Source: CAD feature listing. Evaluate the final solid. Frame: model axes, mm. A direction names the side the tool comes from. Give positions to 0.01 mm unless a question says otherwise; leave off trailing zeros. Loops run counter-clockwise (first coordinate to the right, second up) from the corner with the lowest first, then second, coordinate; pieces in that order, holes last. Notation, with made-up numbers: (-18.75, 40.25) - (-5.75, 40.25) arc R32 ccw to (-5.75, 74.25) - close; hole circle Ø5 at (-40, 25.5). An arc over 180 degrees is marked (long way). Put each result on its own line as item: value.
```python
from build123d import *

# Parameters (mm, degrees)
SKETCH2_W           = 150
SKETCH2_H           = 78
SKETCH2_W_2         = 66
SKETCH2_H_2         = 31
BOSS_EXTRUDE1_DEPTH = 7
FILLET1_R           = 3
SKETCH3_R           = 2.05
CUT_EXTRUDE1_DEPTH  = 10


with BuildPart() as part:
    # Sketch2 → Boss-Extrude1 (new body)
    with BuildSketch(Plane(origin=(0, 0, 0), x_dir=(1, 0, 0), z_dir=(0, 1, 0))):
        Rectangle(SKETCH2_W, SKETCH2_H)
        Rectangle(SKETCH2_W_2, SKETCH2_H_2, mode=Mode.SUBTRACT)
        with BuildLine():
            Line((-39, 10.6), (-36, 10.6))
            ThreePointArc((-36, 10.6), (-33.9, 8.5), (-36, 6.4))
            Line((-36, 6.4), (-39, 6.4))
            ThreePointArc((-39, 6.4), (-41.1, 8.5), (-39, 10.6))
        make_face(mode=Mode.SUBTRACT)
        with BuildLine():
            Line((-39, -10.6), (-36, -10.6))
            ThreePointArc((-36, -10.6), (-33.9, -8.5), (-36, -6.4))
            Line((-36, -6.4), (-39, -6.4))
            ThreePointArc((-39, -6.4), (-41.1, -8.5), (-39, -10.6))
        make_face(mode=Mode.SUBTRACT)
        with BuildLine():
            Line((39, -10.6), (36, -10.6))
            ThreePointArc((36, -10.6), (33.9, -8.5), (36, -6.4))
            Line((36, -6.4), (39, -6.4))
            ThreePointArc((39, -6.4), (41.1, -8.5), (39, -10.6))
        make_face(mode=Mode.SUBTRACT)
        with BuildLine():
            Line((39, 10.6), (36, 10.6))
            ThreePointArc((36, 10.6), (33.9, 8.5), (36, 6.4))
            Line((36, 6.4), (39, 6.4))
            ThreePointArc((39, 6.4), (41.1, 8.5), (39, 10.6))
        make_face(mode=Mode.SUBTRACT)
    extrude(amount=BOSS_EXTRUDE1_DEPTH)

    # Fillet1
    fillet1_edges = [part.edges().sort_by_distance(p)[0] for p in [
        (75, 3.5, 39),
        (-75, 3.5, 39),
        (-75, 3.5, -39),
        (75, 3.5, -39),
    ]]
    fillet(fillet1_edges, radius=FILLET1_R)

    # Sketch3 → Cut-Extrude1 (cut)
    with BuildSketch(Plane(origin=(0, 7, 0), x_dir=(1, 0, 0), z_dir=(0, 1, 0))):
        with Locations(Location((-65, 10, 0), (0, 0, 270))):
            Circle(SKETCH3_R)
        with Locations(Location((-65, 29, 0), (0, 0, 270))):
            Circle(SKETCH3_R)
        with Locations(Location((-65, -10, 0), (0, 0, 270))):
            Circle(SKETCH3_R)
        with Locations(Location((-65, -29, 0), (0, 0, 270))):
            Circle(SKETCH3_R)
        with Locations(Location((65, -29, 0), (0, 0, 270))):
            Circle(SKETCH3_R)
        with Locations(Location((65, -10, 0), (0, 0, 270))):
            Circle(SKETCH3_R)
        with Locations(Location((65, 10, 0), (0, 0, 270))):
            Circle(SKETCH3_R)
        with Locations(Location((65, 29, 0), (0, 0, 270))):
            Circle(SKETCH3_R)
    extrude(amount=-CUT_EXTRUDE1_DEPTH, mode=Mode.SUBTRACT)


solid = part.part
```
1) Material intervals for line 1 along X through (y, z) = (5.75, -29); line 2 along Z through (x, y) = (6, 1); line 3 along X through (y, z) = (6.25, -3), sorted ascending. Write a range as [from, to].
Check result:
line 1: [-75, -67.05], [-62.95, 62.95], [67.05, 75]
line 2: [-39, -15.5], [15.5, 39]
line 3: [-75, -33], [33, 75]
2) Section query C-C, the plane x = -25. Output: boundary loops of the cut face in (y, z).
Check result:
outline: (0, -39) - (7, -39) - (7, -15.5) - (0, -15.5) - close; (0, 15.5) - (7, 15.5) - (7, 39) - (0, 39) - close
3) Pin query (flat end, axial travel): P1, Ø6.5, axis at x = -65, z = 10, coming from the -Y side. Return the tip coordinate at first contact, or that it passes through.
Check result:
P1: y = 0
4) Access query for faces 1 (the flat face through (-33, 3, 0)), 2 (the flat face through (-1, 7, -18)). Directions: +Z, -Z, +X, -X, +Y, -Y. A direction counts if a zero-diameter tool reaches every point of the face in a straight line with its end or side. Return the directions, or none.
Check result:
face 1: +Y, -Y
face 2: +Z, -Z, +X, -X, +Y
5) Section query A-A, the plane x = 65. Output: boundary loops of the cut face in (y, z).
Check result:
outline: (0, -39) - (7, -39) - (7, -31.05) - (0, -31.05) - close; (0, -26.95) - (7, -26.95) - (7, -12.05) - (0, -12.05) - close; (0, -7.95) - (7, -7.95) - (7, 7.95) - (0, 7.95) - close; (0, 12.05) - (7, 12.05) - (7, 26.95) - (0, 26.95) - close; (0, 31.05) - (7, 31.05) - (7, 39) - (0, 39) - close
6) Mould query, pull axis Z, two halves, no side actions, for faces 3 (the flat face through (-75, 3, 1)), 4 (the cylindrical face through (74.1, 3.55, -38.14)), 5 (the flat face through (37, 3, 6.4)). Classes: pulls with the +Z half, pulls with the -Z half, needs draft (parallel to the pull), parting line crosses it, or undercut.
Check result:
face 3: needs draft
face 4: pulls with the -Z half
face 5: undercut
7) Section query B-B, the plane z = 0. Output: boundary loops of the cut face in (x, y), plus the area to 3 significant figures.
Check result:
outline: (-75, 0) - (-33, 0) - (-33, 7) - (-75, 7) - close; (33, 0) - (75, 0) - (75, 7) - (33, 7) - close
area: 588 mm²
8) Section query D-D, the plane y = 3. State how many separate pieces and enclosed holes the cut face has, plus the area to 3 significant figures.
Check result:
separate pieces: 1
enclosed holes: 13
area: 9,430 mm²
